The model under review builds one solid part; all positions refer to its coordinate system, in mm. Coordinates: 2 decimals unless noted, no trailing zeros. Loops run counter-clockwise (first coordinate to the right, second up) from the corner with the lowest first, then second, coordinate; pieces in that order, holes last. Notation, with made-up numbers: (42.25, 41.5) - (81.25, 41.5) arc R17 cw to (81.25, 57.5) - close; hole circle Ø2 at (2.5, -6). An arc over 180 degrees is marked (long way). One line per item, written item: value. Start each with the question number.
1. Insertion check: P1, Ø3, axis at x = -42.6, y = -54.77, coming from the -Z side; P2, Ø4, axis at x = 42.6, y = -54.77, coming from the +Z side (3 decimals); P3, Ø1.6, axis at y = 55.5, z = 2, coming from the +X side. Each pin has a flat end and moves straight along its axis. Give the tip position at first contact, or say it passes through.
2. We need section A-A, the plane x = -38. Give the boundary of the cut face in (y, z) (1 decimal).
3. To check wall thickness, follow line 1 (X direction, y = 50.5, z = 3); line 2 (Y direction, x = 111, z = 0.75); line 3 (X direction, y = 53, z = 1.4) (1 decimal). State the ranges of each line that lie inside material, in increasing order.
4. We need section B-B, the plane y = -37. Give the boundary of the cut face in (x, z) (1 decimal), then the cut area to 3 significant figures.
5. Mouldability with a two-part tool opening along Z and no side actions: class faces 1 (the face through (-10, -52, 3.175)), 2 (the face through (-10, -52, 0)), 3 (the face through (130.314, 57.21, 1.61)) as +Z half, -Z half, draft (parallel to the pull), parting line (faces both ways), or undercut.
6. We need section C-C, the plane z = 2.45. Count the separate pieces of the cut face and the enclosed holes in it, then the cut area to 3 significant figures.
from build123d import *

# Parameters (mm, degrees)
SKETCH_W        = 263.525
SKETCH_H        = 117.475
PAD_DEPTH       = 3.175
SKETCH002_W     = 249.2375
SKETCH002_H     = 103.98125
POCKET_DEPTH    = 3.176
SKETCH003_W     = 14.9225
SKETCH003_H     = 25.4
POCKET001_DEPTH = 3.176
SKETCH001_R     = 1.5494
HOLE_DEPTH      = 3.176
FILLET_R        = 5.08
FILLET001_R     = 1.27


with BuildPart() as part:
    # Sketch → Pad (new body)
    with BuildSketch(Plane.XY):
        Rectangle(SKETCH_W, SKETCH_H)
    extrude(amount=PAD_DEPTH)

    # Sketch002 (on Face6 of Pad) → Pocket (cut, through all)
    with BuildSketch(Plane.XY.offset(3.175)):
        with Locations((0, 0.396875)):
            Rectangle(SKETCH002_W, SKETCH002_H)
    extrude(amount=-POCKET_DEPTH, mode=Mode.SUBTRACT)

    # Sketch003 (on Face5 of Pocket) → Pocket001 (cut, through all)
    with BuildSketch(Plane.XY.offset(3.175)):
        with Locations((82.07375, 46.0375)):
            Rectangle(SKETCH003_W, SKETCH003_H)
    extrude(amount=-POCKET001_DEPTH, mode=Mode.SUBTRACT)

    # Sketch001 (on Face6 of Pad) → Hole (cut, through all)
    with BuildSketch(Plane.XY.offset(3.175)):
        with Locations((-42.597917, 54.76875)):
            Circle(SKETCH001_R)
        with Locations((42.597917, 54.76875)):
            Circle(SKETCH001_R)
        with Locations((42.597917, -54.76875)):
            Circle(SKETCH001_R)
        with Locations((-42.597917, -54.76875)):
            Circle(SKETCH001_R)
        with Locations((-127.79375, -54.76875)):
            Circle(SKETCH001_R)
        with Locations((-127.79375, 54.76875)):
            Circle(SKETCH001_R)
        with Locations((127.79375, 54.76875)):
            Circle(SKETCH001_R)
        with Locations((127.79375, -54.76875)):
            Circle(SKETCH001_R)
    extrude(amount=-HOLE_DEPTH, mode=Mode.SUBTRACT)

    # Fillet
    fillet_edges = [part.edges().sort_by_distance(p)[0] for p in [
        (-131.7625, 58.7375, 1.5875),
        (-131.7625, -58.7375, 1.5875),
        (131.7625, -58.7375, 1.5875),
        (131.7625, 58.7375, 1.5875),
    ]]
    fillet(fillet_edges, radius=FILLET_R)

    # Fillet001
    fillet001_edges = [part.edges().sort_by_distance(p)[0] for p in [
        (-124.61875, 52.3875, 1.5875),
        (124.61875, 52.3875, 1.5875),
        (-124.61875, -51.59375, 1.5875),
        (124.61875, -51.59375, 1.5875),
    ]]
    fillet(fillet001_edges, radius=FILLET001_R)


solid = part.part
Findings below:
1. P1: through
1. P2: z = 3.175
1. P3: x = 131.65
2. outline: (-58.7, 0) - (-51.6, 0) - (-51.6, 3.2) - (-58.7, 3.2) - close; (52.4, 0) - (58.7, 0) - (58.7, 3.2) - (52.4, 3.2) - close
3. line 1: -131.76 to -124.62, 124.62 to 131.76
3. line 2: -58.74 to -51.59, 52.39 to 58.74
3. line 3: -131.8 to 74.6, 89.5 to 131.8
4. outline: (-131.8, 0) - (-124.6, 0) - (-124.6, 3.2) - (-131.8, 3.2) - close; (124.6, 0) - (131.8, 0) - (131.8, 3.2) - (124.6, 3.2) - close
4. area: 45.4 mm2
5. face 1: +Z half
5. face 2: -Z half
5. face 3: draft
6. separate pieces: 1
6. enclosed holes: 8
6. area: 4,870 mm2
